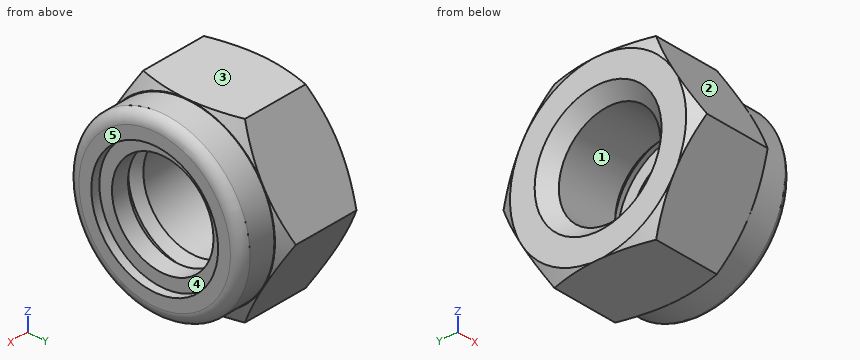
Autodesk Inventor part; units mm, degrees
ref_plane "IP1_XY" through (0, 0, 0) normal (1, 0, 0) x (0, 0, -1)
ref_plane "IP1_YZ" through (0, 0, 0) normal (0, 0, -1) x (0, 1, 0)
ref_plane "IP1_ZX" through (0, 0, 0) normal (0, 1, 0) x (1, 0, 0)
sketch "Sketch_1" plane through (0, 0, 0) normal (0, 0, 1) x (1, 0, 0)
  line L0 (20, 0) -> (0, 0)
  line L1 (0, 0) -> (0, 18)
  line L2 (0, 18) -> (20, 18)
  line L3 (20, 18) -> (20, 10.8)
  line L4 (20, 10.8) -> (18.5, 10.8)
  line L5 (18.5, 10.8) -> (18.5, 8.647)
  line L6 (18.5, 8.647) -> (15.5, 8.647)
  line L7 (15.5, 8.647) -> (15.5, 10.8)
  line L8 (15.5, 10.8) -> (14, 10.8)
  line L9 (14, 10.8) -> (14, 0)
  line L10 (14, 0) -> (0, 0)
revolve "Revolution1" add sketch "Sketch_1" angle 360 about axis through (20, 0, 0) along (-1, 0, 0)
sketch "Sketch_2" plane through (0, 0, 0) normal (1, 0, 0) x (0, 1, 0)
  line L0 (30, 30) -> (-30, 30)
  line L1 (-30, 30) -> (-30, -30)
  line L2 (-30, -30) -> (30, -30)
  line L3 (30, -30) -> (30, 30)
  line L4 (-8.6603, 15) -> (-17.3205, 0)
  line L5 (-17.3205, 0) -> (-8.6603, -15)
  line L6 (-8.6603, -15) -> (8.6603, -15)
  line L7 (8.6603, -15) -> (17.3205, 0)
  line L8 (17.3205, 0) -> (8.6603, 15)
  line L9 (8.6603, 15) -> (-8.6603, 15)
extrude "Extrusion1" cut sketch "Sketch_2" along normal mid plane 42
sketch "Sketch_8" plane through (0, 0, 0) normal (0, 0, 1) x (1, 0, 0)
  line L0 (20, 0) -> (0, 0)
  line L1 (14, 18) -> (14, 14.9)
  line L2 (14, 14.9) -> (20, 14.9)
  line L3 (20, 14.9) -> (20, 18)
  line L4 (20, 18) -> (14, 18)
revolve "Revolution2" cut sketch "Sketch_8" angle 360 about axis through (20, 0, 0) along (1, 0, 0)
sketch "Sketch_4" plane through (0, 0, 0) normal (0, 0, 1) x (1, 0, 0)
  line L0 (14, 0) -> (0, 0)
  line L1 (0, 0) -> (0, 10.8)
  line L2 (0, 10.8) -> (2.153, 8.647)
  line L3 (2.153, 8.647) -> (12.647, 8.647)
  line L4 (12.647, 8.647) -> (14, 10)
  line L5 (14, 10) -> (14, 0)
  line L6 (14, 0) -> (0, 0)
revolve "Revolution3" cut sketch "Sketch_4" angle 360 about axis through (14, 0, 0) along (1, 0, 0)
thread "Thread1"
sketch "Sketch_5" plane through (0, 0, 0) normal (0, 0, 1) x (1, 0, 0)
  line L0 (20, 0) -> (0, 0)
  line L1 (17.8, 15) -> (17.9, 15)
  arc A0 (20, 12.9) -> (17.9, 15) centre (17.9, 12.9) ccw
  line L2 (20, 12.9) -> (20.1, 12.9)
  line L3 (20.1, 12.9) -> (20.1, 22.5)
  line L4 (20.1, 22.5) -> (17.8, 22.5)
  line L5 (17.8, 22.5) -> (17.8, 15)
revolve "Revolution4" cut sketch "Sketch_5" angle 360 about axis through (20, 0, 0) along (1, 0, 0)
sketch "Sketch_6" plane through (0, 0, 0) normal (0, 0, 1) x (1, 0, 0)
  line L0 (20, 0) -> (0, 0)
  line L1 (-1, 15) -> (0, 15)
  line L2 (0, 15) -> (4.3301, 22.5)
  line L3 (4.3301, 22.5) -> (9.6699, 22.5)
  line L4 (9.6699, 22.5) -> (14, 15)
  line L5 (14, 15) -> (15.5, 15)
  line L6 (15.5, 15) -> (15.5, 25.5)
  line L7 (15.5, 25.5) -> (-1, 25.5)
  line L8 (-1, 25.5) -> (-1, 15)
revolve "Revolution5" cut sketch "Sketch_6" angle 360 about axis through (20, 0, 0) along (1, 0, 0)
ref_plane "IP1_XY" through (0, 0, 0) normal (1, 0, 0) x (0, 0, -1)
ref_plane "IP1_YZ" through (0, 0, 0) normal (0, 0, -1) x (0, 1, 0)
ref_plane "IP1_ZX" through (0, 0, 0) normal (0, 1, 0) x (1, 0, 0)
ref_plane "IP2_XY" through (20, 0, 0) normal (1, 0, 0) x (0, 0, -1)
ref_plane "IP2_YZ" through (20, 0, 0) normal (0, 0, -1) x (0, 1, 0)
ref_plane "IP2_ZX" through (20, 0, 0) normal (0, 1, 0) x (1, 0, 0)
properties part number "BN 161 1118811 prevailing torque type hex lock nut M20"
Verification items for the finished model (mm, model axes). Face numbers are marked on the shaded views. A direction names the side the tool comes from. Give positions to 0.01 mm unless a question says otherwise; leave off trailing zeros. Order: outer loops, then holes, each group sorted by start corner. A loop starts at its lowest first (then second) coordinate and runs counter-clockwise, first axis right, second up. Notation, with made-up numbers: (39, 61) -> (76, 61) arc R32 cw to (76, 100) -> close; hole circle Ø1 at (21.25, 12.25). An arc over 180 degrees is marked (long way). One line per item, written item: value.
(1) Sectioned sample at A-A on x = 7. Record the cut outline in (y, z).
Final values:
outline: (-17.32, 0) -> (-8.66, -15) -> (8.66, -15) -> (17.32, 0) -> (8.66, 15) -> (-8.66, 15) -> close; hole circle Ø17.29 at (0, 0)
(2) Draft check along Y on the marked faces 1, 2 and 3. Enter one of: pulls with the +Y half, pulls with the -Y half, needs draft (parallel to the pull), parting line crosses it, or undercut.
Final values:
face 1: undercut
face 2: pulls with the -Y half
face 3: needs draft
(3) Tool access check on the marked faces 4 and 5. Record the directions out of +Z, -Z, +X, -X, +Y, -Y that give a thin tool (end or side, any length) a straight path to the whole face; none if there is none.
Final values:
face 4: +X
face 5: +Z, -Z, +X, +Y, -Y
(4) Scan lines: line 1 along Z through (x, y) = (7.5, 0); line 2 along Z through (x, y) = (14.4, 0); line 3 along X through (y, z) = (-1.5, 9). Record each from-to range of solid material in increasing order. Write a range as [from, to].
Final values:
line 1: [-15, -8.65], [8.65, 15]
line 2: [-14.9, -10.8], [10.8, 14.9]
line 3: [1.68, 13.12], [15.5, 18.5]
(5) Gauge pin test, flat ends, axial feed: pin 1 (11 mm diameter, centred on y = 0, z = 4.5, fed in from +X); pin 2 (10 mm diameter, centred on x = 10.5, z = -6, fed in from -Y); pin 3 (6 mm diameter, centred on x = 17.5, y = -13, fed in from -Z). Record the tip position at first contact, or that the pin passes through.
Final values:
pin 1: x = 18.5
pin 2: y = -16.74
pin 3: z = -11.05
